Here's how the part is built. I have some questions about the finished solid (model axes, mm). A direction names the side the tool comes from. Coordinates: 2 decimals unless noted, no trailing zeros. Write each loop counter-clockwise with the first axis right and the second up, starting at its lowest first coordinate (ties: lowest second). Pieces come first, ordered by that corner, then holes. Notation, with made-up numbers: (72.5, 47.5) -> (91.5, 47.5) arc R31 cw to (91.5, 72.5) -> close; hole circle Ø8 at (-19.5, -12). An arc over 180 degrees is marked (long way). Use a Markdown table: item, result. Add a question column.
Item 1: On a 3-axis mill with a long thin cutter (end or side, diameter ignored), from which of +Z, -Z, +X, -X, +Y, -Y can I reach the whole of each face in a straight line? I mean faces 1 (the flat face through (3, -3, -16)), 2 (the flat face through (-2.4, -25, -13.1)), 3 (the cylindrical face through (-3.47, 14.15, 15.62)). Say none if no direction works.
Item 2: Imagine slicing it at B-B, the plane z = 0. Write out the boundary of the cut face in (x, y).
Item 3: Will these pins go through, and if not, where does the flat tip stop? pin 1 Ø2 at (x, y) = (7, 12) entering from +Z; pin 2 Ø10 at (y, z) = (2, 12) entering from -X; pin 3 Ø3 at (x, y) = (0, 0) entering from -Z.
Item 4: Imagine slicing it at C-C, the plane x = -11. Write out the boundary of the cut face in (y, z), and give its area (3 significant figures).
Item 5: Imagine slicing it at A-A, the plane x = 0. Write out the boundary of the cut face in (y, z), and give its area (3 significant figures).
Item 6: Imagine slicing it at D-D, the plane y = -12.5. Write out the boundary of the cut face in (x, z).
Item 7: If we mould it in two halves opening along X, with no side actions, what happens to faces 4 (the flat face through (3, 3, -16)), 5 (the cylindrical face through (-2.539, 0.042, -19.334)), 6 (the cylindrical face through (0, -2, -16))? For each: pulls with the +X half, pulls with the -X half, needs draft (parallel to the pull), parting line crosses it, or undercut.
Item 8: If I drill on line 1 along Z through (x, y) = (0, -4); line 2 along Y through (x, z) = (0, -15), over which ranges is the centre line in solid material (lowest first)? Write a range as from..to.
```python
from build123d import *

# Parameters (mm, degrees)
SKETCH1_R           = 16
SKETCH1_R_2         = 13.1445
BOSS_EXTRUDE1_DEPTH = 25
SKETCH2_R           = 19.5
SKETCH2_R_2         = 16
BOSS_EXTRUDE2_DEPTH = 3
CUT_EXTRUDE1_REACH  = 21.5
SKETCH3_R           = 2


with BuildPart() as part:
    # Sketch1 → Boss-Extrude1 (new body, symmetric)
    with BuildSketch(Plane(origin=(0, 0, 0), x_dir=(1, 0, 0), z_dir=(0, 1, 0))):
        Circle(SKETCH1_R)
        Circle(SKETCH1_R_2, mode=Mode.SUBTRACT)
    extrude(amount=BOSS_EXTRUDE1_DEPTH, both=True)

    # Sketch2 → Boss-Extrude2 (add, symmetric)
    with BuildSketch(Plane(origin=(0, 0, 0), x_dir=(1, 0, 0), z_dir=(0, 1, 0))):
        Circle(SKETCH2_R)
        Circle(SKETCH2_R_2, mode=Mode.SUBTRACT)
    extrude(amount=BOSS_EXTRUDE2_DEPTH, both=True)

    # Sketch3 → Cut-Extrude1 (cut, up to next)
    with BuildSketch(Plane.XY, mode=Mode.PRIVATE) as cut_extrude1_sk1:
        Circle(SKETCH3_R)
    cut_extrude1_tool1 = extrude(cut_extrude1_sk1.sketch, amount=-CUT_EXTRUDE1_REACH, mode=Mode.PRIVATE) & part.part
    add(cut_extrude1_tool1.solids().sort_by_distance((0, 0, 0))[0], mode=Mode.SUBTRACT)


solid = part.part
```
Ans:
| question | item | result |
|---|---|---|
| 1 | face 1 | -Y |
| 1 | face 2 | +Z, -Z, +X, -X, -Y |
| 1 | face 3 | +Y |
| 2 | outline | (-19.5, -3) -> (-16, -3) -> (-16, -25) -> (-13.14, -25) -> (-13.14, 25) -> (-16, 25) -> (-16, 3) -> (-19.5, 3) -> close; (13.14, -25) -> (16, -25) -> (16, -3) -> (19.5, -3) -> (19.5, 3) -> (16, 3) -> (16, 25) -> (13.14, 25) -> close |
| 3 | pin 1 | stops at z = 14.83 |
| 3 | pin 2 | stops at x = -18.2 |
| 3 | pin 3 | stops at z = 13.06 |
| 4 | outline | (-25, -11.62) -> (-3, -11.62) -> (-3, -16.1) -> (3, -16.1) -> (3, -11.62) -> (25, -11.62) -> (25, -7.2) -> (-25, -7.2) -> close; (-25, 7.2) -> (25, 7.2) -> (25, 11.62) -> (3, 11.62) -> (3, 16.1) -> (-3, 16.1) -> (-3, 11.62) -> (-25, 11.62) -> close |
| 4 | area | 496 mm^2 |
| 5 | outline | (-25, -16) -> (-3, -16) -> (-3, -19.5) -> (-2, -19.5) -> (-2, -13.14) -> (-25, -13.14) -> close; (-25, 13.14) -> (25, 13.14) -> (25, 16) -> (3, 16) -> (3, 19.5) -> (-3, 19.5) -> (-3, 16) -> (-25, 16) -> close; (2, -19.5) -> (3, -19.5) -> (3, -16) -> (25, -16) -> (25, -13.14) -> (2, -13.14) -> close |
| 5 | area | 302 mm^2 |
| 6 | outline | circle Ø32 at (0, 0); hole circle Ø26.29 at (0, 0) |
| 7 | face 4 | needs draft |
| 7 | face 5 | parting line crosses it |
| 7 | face 6 | undercut |
| 8 | line 1 | z = -16..-13.14, 13.14..16 |
| 8 | line 2 | y = -25..-2, 2..25 |
